```python
from build123d import *

# Parameters (mm, degrees)
F1_DEPTH        = 177.8
F1_COPIES_COUNT = 3


# Not quite as in the source:
# - a feature of the source that left no trace in its solid (it failed there, or was rolled back) is left out
# - a pattern or mirror of a feature is missing from the dataset's text; its kind, count and spacing are read off the source's solid


with BuildPart() as f1:
    # F0 (on Top) → F1 (new body)
    with BuildSketch(Plane.XY):
        with BuildLine():
            ThreePointArc((75.565, 0), (355.6, 280.035), (635.635, 0))
            Line((635.635, 0), (711.2, 0))
            ThreePointArc((711.2, 0), (355.6, 355.6), (0, 0))
            Line((0, 0), (75.565, 0))
        make_face()
        with BuildLine():
            Line((711.2, 0), (635.635, 0))
            ThreePointArc((635.635, 0), (355.6, -280.035), (75.565, 0))
            Line((75.565, 0), (0, 0))
            ThreePointArc((0, 0), (355.6, -355.6), (711.2, 0))
        make_face()
        with BuildLine():
            Line((711.2, -762), (711.2, 0))
            ThreePointArc((711.2, 0), (355.6, -355.6), (0, 0))
            Line((0, 0), (0, -762))
            ThreePointArc((0, -762), (355.6, -406.4), (711.2, -762))
        make_face()
        with BuildLine():
            ThreePointArc((0, -762), (355.6, -1117.6), (711.2, -762))
            Line((711.2, -762), (635.635, -762))
            ThreePointArc((635.635, -762), (355.6, -1042.035), (75.565, -762))
            Line((75.565, -762), (0, -762))
        make_face()
        with BuildLine():
            Line((635.635, -762), (711.2, -762))
            ThreePointArc((711.2, -762), (355.6, -406.4), (0, -762))
            Line((0, -762), (75.565, -762))
            ThreePointArc((75.565, -762), (355.6, -481.965), (635.635, -762))
        make_face()
    extrude(amount=F1_DEPTH)

    # F1_copies: F1 ×3 about axis
    f1_copies_axis = Axis((355.6, -762, 0), (0, 0, 1))


with BuildPart() as f1_1:
    add(f1.part)
    for i in range(1, F1_COPIES_COUNT):
        add(f1.part.rotate(f1_copies_axis, i * 360 / F1_COPIES_COUNT))


solid = f1_1.part
```
The model under review builds one solid part; all positions refer to its coordinate system, in mm. A direction names the side the tool comes from. Round coordinates to 2 decimals unless told otherwise and drop trailing zeros. Write each loop counter-clockwise with the first axis right and the second up, starting at its lowest first coordinate (ties: lowest second). Pieces come first, ordered by that corner, then holes.
(1) Machinability: for faces 1 (the cylindrical face through (363.419, 355.514, 87.655)), 2 (the flat face through (593.281, -1309.837, 87.655)), 3 (the flat face through (711.2, -282, 88)), which of the approach directions +Z, -Z, +X, -X, +Y, -Y give a long, thin tool a straight path to every point of the face, cutting with its end or side? Answer none if there is none.
(2) Insertion check: pin 1 (3 mm diameter, centred on y = -933, z = 59, fed in from -X); pin 2 (5 mm diameter, centred on y = -378.5, z = 49, fed in from +X); pin 3 (1.5 mm diameter, centred on x = 399, z = 148.5, fed in from -Y). Each pin has a flat end and moves straight along its axis. Give the tip position at first contact, or say it passes through.
(3) Mouldability with a two-part tool opening along X and no side actions: class faces 4 (the flat face through (0, -274, 88)), 5 (the flat face through (57, -845, 177.8)), 6 (the cylindrical face through (622.704, -84.115, 87.655)) as +X half, -X half, draft (parallel to the pull), parting line (faces both ways), or undercut.
(4) Wall thickness on L1, parallel to Y at x = 355.6, z = 94 (3 decimals); L2, parallel to X at y = 0, z = 117 (3 decimals); L3, parallel to X at y = -1392.5, z = 100: over which ranges is each line inside the solid? List them lowest first.
(5) We need section D-D on z = 103. Give the boundary of the cut face in (x, y) (3 decimals), and give its area (3 significant figures).
(6) We need section B-B on y = -1143. Give the boundary of the cut face in (x, z).
(7) We need section A-A on y = -762. Give the boundary of the cut face in (x, z) (3 decimals), and give its area (3 significant figures).
(8) We need section C-C on x = 159. Give the boundary of the cut face in (y, z), and give its area (3 significant figures).
Findings below:
1. face 1: +Z, -Z, +Y
1. face 2: +Z, -Z, -Y
1. face 3: +Z, -Z, +X, +Y
2. pin 1: stops at x = -592.37
2. pin 2: stops at x = 711.2
2. pin 3: stops at y = -1198.1
3. face 4: -X half
3. face 5: draft
3. face 6: undercut
4. L1: y = -1172.612 to -1042.035, -481.965 to -280.035, 280.035 to 355.6
4. L2: x = 0 to 75.565, 635.635 to 711.2
4. L3: x = -557.69 to -431.47, -177.15 to -25.26, 736.46 to 888.35, 1142.67 to 1268.89
5. outline: (-482.111, -835.041) arc R355.6 ccw to (-126.511, -1450.959) - (355.6, -1172.612) - (837.711, -1450.959) arc R355.6 ccw to (1193.311, -835.041) - (711.2, -556.694) - (711.2, 0) arc R355.6 ccw to (0, 0) - (0, -556.694) - close; hole circle Ø560.07 at (-304.311, -1143); hole circle Ø560.07 at (355.6, -762); hole circle Ø560.07 at (355.6, 0); hole circle Ø560.07 at (1015.511, -1143)
5. area: 1,020,000 mm2
6. outline: (-659.91, 0) - (-584.35, 0) - (-584.35, 177.8) - (-659.91, 177.8) - close; (-24.28, 0) - (735.48, 0) - (735.48, 177.8) - (-24.28, 177.8) - close; (1295.55, 0) - (1371.11, 0) - (1371.11, 177.8) - (1295.55, 177.8) - close
7. outline: (-355.6, 0) - (75.565, 0) - (75.565, 177.8) - (-355.6, 177.8) - close; (635.635, 0) - (1066.8, 0) - (1066.8, 177.8) - (635.635, 177.8) - close
7. area: 153,000 mm2
8. outline: (-1286.12, 0) - (-961.42, 0) - (-961.42, 177.8) - (-1286.12, 177.8) - close; (-562.58, 0) - (-199.42, 0) - (-199.42, 177.8) - (-562.58, 177.8) - close; (199.42, 0) - (296.31, 0) - (296.31, 177.8) - (199.42, 177.8) - close
8. area: 140,000 mm2
